The model under review builds one solid part; all positions refer to its coordinate system, in mm. A direction names the side the tool comes from. Coordinates: 2 decimals unless noted, no trailing zeros. Write each loop counter-clockwise with the first axis right and the second up, starting at its lowest first coordinate (ties: lowest second). Pieces come first, ordered by that corner, then holes. Notation, with made-up numbers: (44, 65) - (48, 65) arc R27 cw to (48, 84) - close; hole circle Ø2 at (33, 38.25). An arc over 180 degrees is marked (long way). Return JSON: item names as keys, results as strings. Group by question number.
(1) For pin 1 Ø1.5 at (x, y) = (-25, 36.5) entering from +Z; pin 2 Ø5 at (y, z) = (4, -97) entering from +X; pin 3 Ø4 at (y, z) = (19.5, 119) entering from -X, all flat-tipped, find the tip position at first contact; note any pin that passes through.
(2) We need section B-B on x = 7.5. State the section outline as (y, z) points, then the cut area to 3 significant figures.
(3) Draft analysis for pull direction Z (two halves, no side actions). For faces 4 (the face through (-17.82, 15.9, -156.92)), 5 (the face through (13.13, 27.2, -157.25)), 6 (the face through (-19.92, 21.53, -51.3)), state which applies: released by +Z, released by -Z, zero draft, split by the parting line, or undercut.
(4) We need section A-A on z = 99. State the section outline as (x, y) points, then the cut area to 3 significant figures.
(5) Tool access review of faces 1 (the face through (-15.75, 16.58, -154.79)), 2 (the face through (7.67, 24.28, 157.2)), 3 (the face through (-19.92, 21.53, 94.75)): name each direction out of +Z, -Z, +X, -X, +Y, -Y from which nothing blocks a thin tool from reaching the whole face with its end or side.
(6) We need section D-D on z = 2. State the section outline as (x, y) points, then the cut area to 3 significant figures.
(7) We need section C-C on y = 24. Give the number of separate pieces and of enclosed holes in the cut face, then the cut area to 3 significant figures.
(8) To check wall thickness, follow L1, parallel to Z at x = -6, y = 45; L2, parallel to Z at x = -26.5, y = 53.5; L3, parallel to X at y = 35.5, z = 9. State the ranges of each line that lie inside material, in increasing order. Write a range as from..to.
Autodesk Inventor part; units mm, degrees
ref_plane "YZ Plane" through (0, 0, 0) normal (1, 0, 0) x (0, 1, 0)
ref_plane "XZ Plane" through (0, 0, 0) normal (0, 1, 0) x (-1, 0, 0)
ref_plane "XY Plane" through (0, 0, 0) normal (0, 0, 1) x (1, 0, 0)
ref_plane "Work Plane1" through (231.2168, -695.9876, -158.75) normal (0, 0, 1) x (-0.9997801, -0.0209692, 0)
sketch "Sketch1" plane through (231.2168, -695.9876, -158.75) normal (0, 0, 1) x (-0.9997801, -0.0209692, 0)
  line L0 (191.5805, -690.6559) -> (218.9069, -682.3014)
  line L1 (218.9069, -682.3014) -> (241.1856, -755.1718)
  line L2 (241.1856, -755.1718) -> (213.8592, -763.5264)
  line L3 (213.8592, -763.5264) -> (191.5805, -690.6559)
  arc A0 (211.507, -928.635) -> (222.8439, -923.2276) centre (216.7713, -925.0841) ccw
  line L4 (203.7328, -860.718) -> (222.8439, -923.2276)
  arc A1 (207.9488, -852.7889) -> (203.7328, -860.718) centre (209.8053, -858.8615) ccw
  line L5 (232.2389, -845.3627) -> (207.9488, -852.7889)
  arc A2 (240.168, -849.5787) -> (232.2389, -845.3627) centre (234.0955, -851.4352) ccw
  line L6 (288.8094, -1008.6774) -> (240.168, -849.5787)
  arc A3 (288.8094, -1008.6774) -> (289.6175, -1010.3717) centre (294.8819, -1006.8208) ccw
  line L7 (308.7826, -1038.7851) -> (289.6175, -1010.3717)
  arc A4 (308.7826, -1038.7851) -> (317.5979, -1040.4986) centre (314.047, -1035.2342) ccw
  line L8 (596.6104, -852.3023) -> (317.5979, -1040.4986)
  line L9 (312.5405, -431.1512) -> (596.6104, -852.3023)
  line L10 (95.3316, -577.6604) -> (312.5405, -431.1512)
  arc A5 (95.3316, -577.6604) -> (92.8099, -584.7814) centre (98.8825, -582.9248) ccw
  line L11 (186.4087, -890.9291) -> (92.8099, -584.7814)
  arc A6 (186.4087, -890.9291) -> (187.2168, -892.6234) centre (192.4812, -889.0725) ccw
  line L12 (211.507, -928.635) -> (187.2168, -892.6234)
  line L13 (151.3976, -689.5372) -> (192.5934, -824.2828)
  arc A7 (155.6135, -681.6081) -> (151.3976, -689.5372) centre (157.4701, -687.6806) ccw
  line L14 (179.9037, -674.1818) -> (155.6135, -681.6081)
  arc A8 (187.8328, -678.3978) -> (179.9037, -674.1818) centre (181.7602, -680.2544) ccw
  line L15 (229.0286, -813.1435) -> (187.8328, -678.3978)
  arc A9 (224.8127, -821.0726) -> (229.0286, -813.1435) centre (222.9561, -815) ccw
  line L16 (200.5225, -828.4988) -> (224.8127, -821.0726)
  arc A10 (192.5934, -824.2828) -> (200.5225, -828.4988) centre (198.666, -822.4263) ccw
  arc A11 (140.2582, -653.102) -> (148.1873, -657.3179) centre (146.3307, -651.2454) ccw
  line L17 (122.5952, -595.3289) -> (140.2582, -653.102)
  arc A12 (125.1168, -588.2079) -> (122.5952, -595.3289) centre (128.6677, -593.4723) ccw
  line L18 (147.1366, -573.3554) -> (125.1168, -588.2079)
  arc A13 (156.76, -576.7633) -> (147.1366, -573.3554) centre (150.6874, -578.6198) ccw
  line L19 (176.6934, -641.9626) -> (156.76, -576.7633)
  arc A14 (172.4774, -649.8917) -> (176.6934, -641.9626) centre (170.6209, -643.8192) ccw
  line L20 (148.1873, -657.3179) -> (172.4774, -649.8917)
  line L21 (440.6793, -731.4527) -> (242.0503, -738.1789)
  arc A15 (235.844, -729.7287) -> (242.0503, -738.1789) centre (241.8354, -731.8326) ccw
  line L22 (235.844, -729.7287) -> (312.2467, -512.1467)
  arc A16 (323.7318, -511.066) -> (312.2467, -512.1467) centre (318.238, -514.2505) ccw
  line L23 (323.7318, -511.066) -> (445.9582, -721.9218)
  arc A17 (440.6793, -731.4527) -> (445.9582, -721.9218) centre (440.4644, -725.1063) ccw
  line L24 (293.699, -488.3023) -> (226.6453, -679.2602)
  arc A18 (214.5814, -679.0129) -> (226.6453, -679.2602) centre (220.6539, -677.1564) ccw
  line L25 (214.5814, -679.0129) -> (177.6445, -558.1977)
  arc A19 (180.1661, -551.0767) -> (177.6445, -558.1977) centre (183.717, -556.3411) ccw
  line L26 (180.1661, -551.0767) -> (284.1568, -480.9341)
  arc A20 (293.699, -488.3023) -> (284.1568, -480.9341) centre (287.7077, -486.1985) ccw
  line L27 (338.9686, -980.6315) -> (474.0479, -788.3553)
  arc A21 (484.7375, -788.821) -> (474.0479, -788.3553) centre (479.2438, -792.0056) ccw
  line L28 (484.7375, -788.821) -> (526.8957, -861.5491)
  arc A22 (524.9528, -869.998) -> (526.8957, -861.5491) centre (521.4019, -864.7336) ccw
  line L29 (524.9528, -869.998) -> (347.7154, -989.5462)
  arc A23 (338.9686, -980.6315) -> (347.7154, -989.5462) centre (344.1645, -984.2818) ccw
  line L30 (303.3396, -969.3278) -> (242.8789, -771.57)
  arc A24 (248.7366, -763.3671) -> (242.8789, -771.57) centre (248.9515, -769.7134) ccw
  line L31 (248.7366, -763.3671) -> (452.9866, -756.4505)
  arc A25 (458.3974, -766.4471) -> (452.9866, -756.4505) centre (453.2015, -762.7968) ccw
  line L32 (458.3974, -766.4471) -> (314.608, -971.1215)
  arc A26 (303.3396, -969.3278) -> (314.608, -971.1215) centre (309.4121, -967.4712) ccw
  line L33 (215.2197, -740.1923) -> (205.7566, -709.24)
  line L34 (210.4881, -724.7162) -> (230.0462, -718.7366) construction
  point P0 (216.5716, -700.683)
  dimension "d0" = 76.2
  dimension "d27" = 28.575
extrude "Plate1" add sketch "Sketch1" along normal blind 3.048 contours L0 A18 L1 L2 L3 | L0 L1 A18
sketch "Sketch2" plane through (-4.8448, -19.3786, -152.654) normal (-0.9499637, -0.3123604, 0) x (0.3123604, -0.9499637, 0)
  line L0 (-76.2, 0) -> (0, 0)
  line L1 (0, 0) -> (0, 311.404)
  line L2 (0, 311.404) -> (-76.2, 311.404)
  line L3 (-76.2, 311.404) -> (-76.2, 0)
edge flange "Flange1" height 317.5 angle 90 thickness 3.048 bend radius 3.048 thickness toward (-0.9499637, -0.3123604, 0) relief tear relief width 3.048 relief depth 1.524 edges at (-13.8502, 17.7671, -155.702) wall of the first edge with corners at (-28.6466, 53.0087, -152.654) (-4.8448, -19.3786, -152.654) (-4.8448, -19.3786, 158.75) (-28.6466, 53.0087, 158.75)
bend "Bend1"
corner "Corner1"
sketch "Sketch3" plane through (-7.7403, -20.3306, 155.702) normal (0, 0, 1) x (1, 0, 0)
  line L0 (-23.8019, 72.3872) -> (0, 0)
  line L1 (0, 0) -> (27.1452, 8.9257)
  line L2 (27.1452, 8.9257) -> (3.3434, 81.3129)
  line L3 (3.3434, 81.3129) -> (-23.8019, 72.3872)
edge flange "Flange2" height 28.575 angle 90 thickness 3.048 bend radius 3.048 thickness toward (0, 0, 1) relief tear relief width 3.048 relief depth 1.524 edges at (-16.7457, 16.815, 158.75) wall of the first edge with corners at (-31.5421, 52.0566, 155.702) (-7.7403, -20.3306, 155.702) (19.4049, -11.4049, 155.702) (-4.3969, 60.9823, 155.702)
bend "Bend2"
corner "Corner2"
sketch "Sketch4" plane through (-31.5421, 52.0566, 152.654) normal (-0.9499637, -0.3123604, 0) x (0, 0, -1)
  line L0 (-6.096, 80.617) -> (-6.096, -4.417)
  line L1 (-6.096, 38.1) -> (311.404, 38.1) construction
  line L2 (311.404, 74.4136) -> (311.404, 1.7864)
  circle A0 centre (44.704, 38.1) radius 31.75
  circle A1 centre (114.554, 38.1) radius 38.1
  circle A2 centre (190.754, 38.1) radius 38.1
  circle A3 centre (260.604, 38.1) radius 31.75
  circle A4 centre (44.704, 38.1) radius 16.2087 construction
  circle A5 centre (260.604, 38.1) radius 16.2087 construction
  circle A6 centre (44.704, 38.1) radius 14.2875
  circle A7 centre (114.554, 38.1) radius 14.2875
  circle A8 centre (190.754, 38.1) radius 14.2875
  circle A9 centre (260.604, 38.1) radius 14.2875
  line L3 (-6.096, 0) -> (-6.096, 76.2)
  line L4 (311.404, 0) -> (311.404, 76.2)
  line L5 (44.704, 38.1) -> (-6.096, 38.1) construction
  line L6 (260.604, 38.1) -> (311.404, 38.1) construction
  dimension "d22" = 28.575
  dimension "d23" = 63.5
  dimension "d28" = 76.2
extrude "Cut1" cut sketch "Sketch4" against normal blind 3.048 contours A6 | A7 | A8 | A9
equation "\"d25\" = Thickness"
equation "\"d1\" = Thickness"
equation "\"d2\" = BendReliefWidth"
equation "\"d3\" = BendReliefDepth"
equation "\"d4\" = MinimumRemnant"
equation "\"d5\" = TransitionRadius"
equation "\"d8\" = BendRadius"
equation "\"d9\" = CornerReliefSize"
equation "\"d10\" = GapSize"
equation "\"d11\" = JacobiRadiusSize"
equation "\"d12\" = BendReliefWidth"
equation "\"d13\" = BendReliefDepth"
equation "\"d14\" = MinimumRemnant"
equation "\"d15\" = TransitionRadius"
equation "\"d18\" = BendRadius"
equation "\"d19\" = CornerReliefSize"
equation "\"d20\" = GapSize"
equation "\"d21\" = JacobiRadiusSize"
equation "\"BendRadius\" = Thickness"
equation "\"BendReliefWidth\" = Thickness"
equation "\"BendReliefDepth\" = 0.5 * Thickness"
equation "\"CornerReliefSize\" = 4 * Thickness"
equation "\"MinimumRemnant\" = 2 * Thickness"
equation "\"TransitionRadius\" = BendRadius"
equation "\"JacobiRadiusSize\" = BendRadius"
equation "\"GapSize\" = Thickness"
properties part number "GearBracket"
Ans:
{
 "1": {"pin 1": "z = 157.26", "pin 2": "x = -11.71", "pin 3": "through"},
 "2": {"outline": "(-15.32, -158.75) - (44.32, -158.75) - (44.32, -155.7) - (-15.32, -155.7) - close; (-15.32, 155.7) - (24.8, 155.7) - (24.8, 158.75) - (-15.32, 158.75) - close", "area": "304 mm²"},
 "3": {"face 4": "released by -Z", "face 5": "zero draft", "face 6": "undercut"},
 "4": {"outline": "(-31.54, 52.06) - (-23.12, 26.44) - (-20.22, 27.39) - (-28.65, 53.01) - close; (-16.16, 5.28) - (-7.74, -20.33) - (-4.84, -19.38) - (-13.27, 6.24) - close", "area": "164 mm²"},
 "5": {"face 1": "+X, +Y", "face 2": "+Z, +X, +Y", "face 3": "none"},
 "6": {"outline": "(-31.54, 52.06) - (-7.74, -20.33) - (-4.84, -19.38) - (-28.65, 53.01) - close", "area": "232 mm²"},
 "7": {"separate pieces": "5", "enclosed holes": "0", "area": "887 mm²"},
 "8": {"L1": "-158.75..-155.7, 155.7..158.75", "L2": "-158.69..-155.58, 155.58..158.69", "L3": "-26.1..-22.89"}
}
